```python
from build123d import *

# Parameters (mm, degrees)
BOSS_EXTRUDE1_DEPTH = 2.3
SKETCH3_W           = 10
SKETCH3_H           = 8
BOSS_EXTRUDE2_DEPTH = 0.6


with BuildPart() as part:
    # Sketch2 → Boss-Extrude1 (new body, symmetric)
    with BuildSketch(Plane(origin=(0, 0, 0), x_dir=(1, 0, 0), z_dir=(0, 1, 0))):
        with BuildLine():
            Line((0, 4), (1.2, 4))
            ThreePointArc((1.2, 4), (2.2, 0), (1.2, -4))
            Line((1.2, -4), (0, -4))
            ThreePointArc((0, -4), (1, 0), (0, 4))
        make_face()
    extrude(amount=BOSS_EXTRUDE1_DEPTH, both=True)

    # Sketch3 → Boss-Extrude2 (add, symmetric)
    with BuildSketch(Plane(origin=(0, 0, 0), x_dir=(1, 0, 0), z_dir=(0, 1, 0))):
        with Locations((-3.8, 0)):
            Rectangle(SKETCH3_W, SKETCH3_H)
    extrude(amount=BOSS_EXTRUDE2_DEPTH, both=True)


solid = part.part
```
Source: CAD feature listing. Evaluate the final solid. Frame: model axes, mm. A direction names the side the tool comes from. Round coordinates to 2 decimals unless told otherwise and drop trailing zeros. Loops run counter-clockwise (first coordinate to the right, second up) from the corner with the lowest first, then second, coordinate; pieces in that order, holes last. Notation, with made-up numbers: M 11,55 L 36,55 A24 cw 36,92 Z; hole C -31,64 d11. An arc over 180 degrees is marked long. Put each result on its own line as item: value.
(1) Section A-A, the plane z = 0. Return loops of the section in (x, y).
Solutions:
outline: M -8.8,-0.6 L 1,-0.6 L 1,-2.3 L 2.2,-2.3 L 2.2,2.3 L 1,2.3 L 1,0.6 L -8.8,0.6 Z
(2) Ray query, line 1 (Y direction, x = -7.25, z = 3); line 2 (X direction, y = 1.45, z = 3); line 3 (X direction, y = 0.85, z = -2.5). Return the intervals inside material, ascending. Write a range as [from, to].
Solutions:
line 1: [-0.6, 0.6]
line 2: [0.45, 1.65]
line 3: [0.62, 1.82]
(3) First-contact query: pin 1 (2 mm diameter, centred on x = -5.5, y = -1.5, fed in from -Z); pin 2 (1.5 mm diameter, centred on y = 1, z = -1.5, fed in from +X); pin 3 (1.5 mm diameter, centred on y = 1.5, z = -2.5, fed in from -X); pin 4 (2.5 mm diameter, centred on x = -5.5, z = -0.5, fed in from -Y). Flat tips, straight axial feed; report the tip coordinate or a pass-through.
Solutions:
pin 1: z = -4
pin 2: x = 2.17
pin 3: x = 0.35
pin 4: y = -0.6
(4) Access query for faces 1 (the face through (1, 1, 0)), 2 (the face through (1.4, -2.3, -0.1)), 3 (the face through (1, -1, 0)). Directions: +Z, -Z, +X, -X, +Y, -Y. A direction counts if a zero-diameter tool reaches every point of the face in a straight line with its end or side. Return the directions, or none.
Solutions:
face 1: -X, +Y
face 2: +Z, -Z, +X, -X, -Y
face 3: -X, -Y
(5) Section C-C, the plane y = -1.15. Return loops of the section in (x, z).
Solutions:
outline: M 0,-4 L 1.2,-4 A8.5 ccw 1.2,4 L 0,4 A8.5 cw Z
(6) Section D-D, the plane z = 3.25. Return loops of the section in (x, y), and give its area (3 significant figures).
Solutions:
outline: M -8.8,-0.6 L 0.35,-0.6 L 0.35,-2.3 L 1.55,-2.3 L 1.55,2.3 L 0.35,2.3 L 0.35,0.6 L -8.8,0.6 Z
area: 16.5 mm²
(7) Section B-B, the plane x = 0.25. Return loops of the section in (y, z).
Solutions:
outline: M -2.3,-4 L 2.3,-4 L 2.3,-3.49 L 0.6,-3.49 L 0.6,3.49 L 2.3,3.49 L 2.3,4 L -2.3,4 L -2.3,3.49 L -0.6,3.49 L -0.6,-3.49 L -2.3,-3.49 Z
